```python
from build123d import *

# Parameters (mm, degrees)
SKETCH1_W           = 50
SKETCH1_H           = 50
SKETCH1_R           = 2
SKETCH1_W_2         = 16
SKETCH1_H_2         = 11
BOSS_EXTRUDE1_DEPTH = 2
SKETCH2_W           = 50
SKETCH2_H           = 50
SKETCH2_R           = 3.1
SKETCH2_W_2         = 16
SKETCH2_H_2         = 11
BOSS_EXTRUDE2_DEPTH = 18
FILLET1_R           = 3


with BuildPart() as part:
    # Sketch1 → Boss-Extrude1 (new body)
    with BuildSketch(Plane.XY):
        Rectangle(SKETCH1_W, SKETCH1_H)
        with Locations((-11.8, 11.8)):
            Circle(SKETCH1_R, mode=Mode.SUBTRACT)
        with Locations((-11.8, -11.8)):
            Circle(SKETCH1_R, mode=Mode.SUBTRACT)
        with Locations((11.8, -11.8)):
            Circle(SKETCH1_R, mode=Mode.SUBTRACT)
        with Locations((11.8, 11.8)):
            Circle(SKETCH1_R, mode=Mode.SUBTRACT)
        with Locations((0, -11.8)):
            Rectangle(SKETCH1_W_2, SKETCH1_H_2, mode=Mode.SUBTRACT)
    extrude(amount=BOSS_EXTRUDE1_DEPTH)

    # Sketch2 → Boss-Extrude2 (add)
    with BuildSketch(Plane(origin=(0, 0, 0), x_dir=(-1, 0, 0), z_dir=(0, 0, -1))):
        Rectangle(SKETCH2_W, SKETCH2_H)
        with Locations((-11.8, -11.8)):
            Circle(SKETCH2_R, mode=Mode.SUBTRACT)
        with Locations((11.8, -11.8)):
            Circle(SKETCH2_R, mode=Mode.SUBTRACT)
        with Locations((11.8, 11.8)):
            Circle(SKETCH2_R, mode=Mode.SUBTRACT)
        with Locations((-11.8, 11.8)):
            Circle(SKETCH2_R, mode=Mode.SUBTRACT)
        with Locations((0, -11.8)):
            Rectangle(SKETCH2_W_2, SKETCH2_H_2, mode=Mode.SUBTRACT)
    extrude(amount=BOSS_EXTRUDE2_DEPTH)

    # Fillet1
    fillet1_edges = [part.edges().sort_by_distance(p)[0] for p in [
        (25, -25, -8),
        (-25, -25, -8),
        (-25, 25, -8),
        (25, 25, -8),
    ]]
    fillet(fillet1_edges, radius=FILLET1_R)


solid = part.part
```
Geometry check sheet. Reference: the model listing, model coordinates, mm. A direction names the side the tool comes from. Coordinates: 2 decimals unless noted, no trailing zeros. Write each loop counter-clockwise with the first axis right and the second up, starting at its lowest first coordinate (ties: lowest second). Pieces come first, ordered by that corner, then holes. Notation, with made-up numbers: M 47.5,89 L 68.5,89 A18 cw 68.5,117 Z; hole C -36,-20.5 d4. An arc over 180 degrees is marked long. One line per item, written item: value. Start each with the question number.
(1) Sectioned sample at A-A, the plane y = 11.8. Enter the section's corners in (x, z), and give its area (3 significant figures).
(2) Depth check by flat-ended pin: pin 1 (4.5 mm diameter, centred on x = 11.8, y = 11.8, fed in from -Z); pin 2 (2.5 mm diameter, centred on x = -11.8, y = -11.8, fed in from +Z). Enter the tip coordinate at first touch or a pass-through.
(3) Sectioned sample at D-D, the plane y = -11.8. Enter the section's corners in (x, z), and give its area (3 significant figures).
(4) Sectioned sample at B-B, the plane z = -12. Enter the section's corners in (x, y).
(5) Tool access check on faces 1 (the face through (0, -25, -8)), 2 (the face through (8, -12, -8)), 3 (the face through (12.204, 14.874, -8.874)). Record the directions out of +Z, -Z, +X, -X, +Y, -Y that give a thin tool (end or side, any length) a straight path to the whole face; none if there is none.
(6) Scan lines: line 1 along Y through (x, z) = (11.8, -4.75); line 2 along Y through (x, z) = (11.8, 1.4); line 3 along Y through (x, z) = (1.5, -6). Record each from-to range of solid material in increasing order. Write a range as [from, to].
(7) Release check for a two-part mould opening along X. For faces 4 (the face through (-24.1, -24.14, -8.14)), 5 (the face through (0, 25, -8)), 6 (the face through (14, -12, 0)) record: released by +X, released by -X, zero draft, split by the parting line, or undercut.
Filled sheet:
1. outline: M -25,-18 L -14.9,-18 L -14.9,0 L -13.8,0 L -13.8,2 L -25,2 Z; M -9.8,0 L -8.7,0 L -8.7,-18 L 8.7,-18 L 8.7,0 L 9.8,0 L 9.8,2 L -9.8,2 Z; M 13.8,0 L 14.9,0 L 14.9,-18 L 25,-18 L 25,2 L 13.8,2 Z
1. area: 761 mm²
2. pin 1: z = 0
2. pin 2: through
3. outline: M -25,-18 L -14.9,-18 L -14.9,0 L -13.8,0 L -13.8,2 L -25,2 Z; M -9.8,0 L -8.7,0 L -8.7,-18 L -8,-18 L -8,2 L -9.8,2 Z; M 8,-18 L 8.7,-18 L 8.7,0 L 9.8,0 L 9.8,2 L 8,2 Z; M 13.8,0 L 14.9,0 L 14.9,-18 L 25,-18 L 25,2 L 13.8,2 Z
3. area: 441 mm²
4. outline: M -25,-22 A3 ccw -22,-25 L 22,-25 A3 ccw 25,-22 L 25,22 A3 ccw 22,25 L -22,25 A3 ccw -25,22 Z; hole C -11.8,-11.8 d6.2; hole C -11.8,11.8 d6.2; hole M -8,-17.3 L 8,-17.3 L 8,-6.3 L -8,-6.3 Z; hole C 11.8,-11.8 d6.2; hole C 11.8,11.8 d6.2
5. face 1: +Z, -Z, +X, -X, -Y
5. face 2: +Z, -Z
5. face 3: -Z
6. line 1: [-25, -14.9], [-8.7, 8.7], [14.9, 25]
6. line 2: [-25, -13.8], [-9.8, 9.8], [13.8, 25]
6. line 3: [-25, -17.3], [-6.3, 25]
7. face 4: released by -X
7. face 5: zero draft
7. face 6: undercut
